Part print with two shaded views. Sizes in mm from the minimum x, y, z corner. A direction names the side the tool comes from. Round coordinates to 2 decimals unless told otherwise and drop trailing zeros. Loops run counter-clockwise (first coordinate to the right, second up) from the corner with the lowest first, then second, coordinate; pieces in that order, holes last. Notation, with made-up numbers: (17, 7) - (66, 7) arc R9 cw to (66, 22) - close; hole circle Ø3 at (85.25, -0.75). An arc over 180 degrees is marked (long way). Use a Markdown table: item, result.
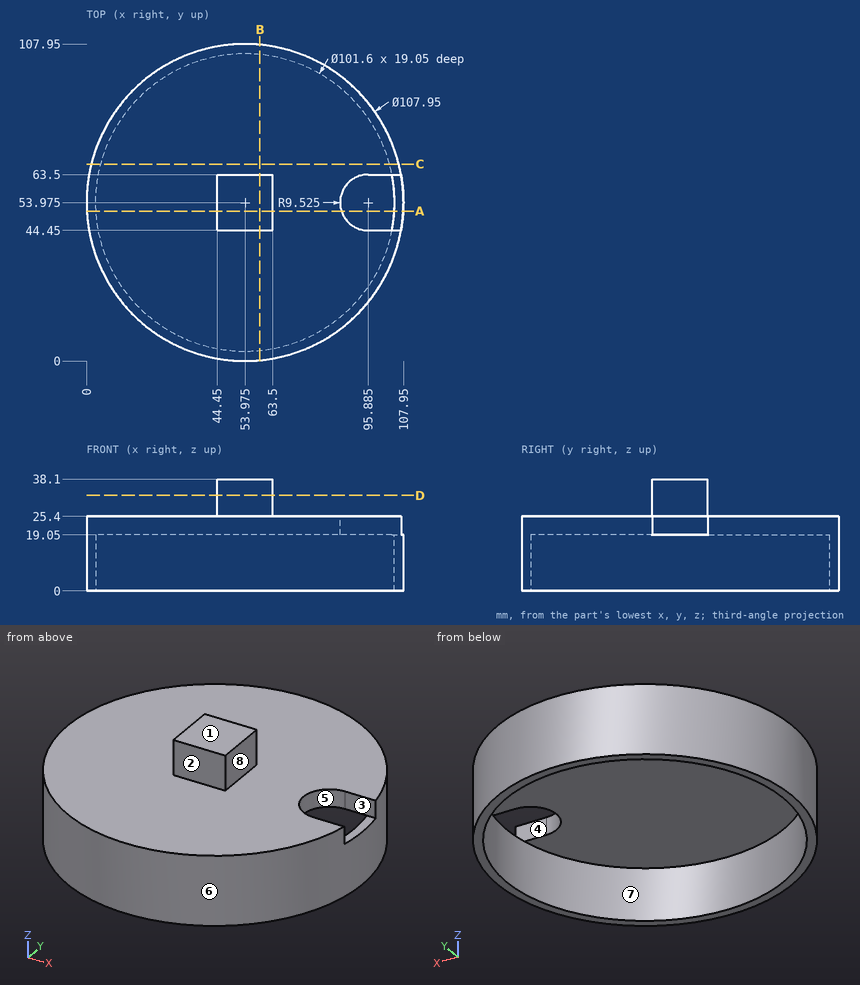
Q1. Which spindle directions (+Z, -Z, +X, -X, +Y, -Y) get a long thin tool onto all of the face, cutting with end or side? Do the marked faces 4, 5, 6, 7 and 8. Say none if no direction does.
Results found:
| item | result |
|---|---|
| face 4 | +Z, +X |
| face 5 | +Z, -Z, +X |
| face 6 | +Z, -Z |
| face 7 | -Z |
| face 8 | +Z, +X, +Y, -Y |
Q2. Cut at A-A, the plane y = 51. List the corners of the cut face in (x, z).
Results found:
| item | result |
|---|---|
| outline | (0.08, 0) - (3.26, 0) - (3.26, 19.05) - (86.84, 19.05) - (86.84, 25.4) - (63.5, 25.4) - (63.5, 38.1) - (44.45, 38.1) - (44.45, 25.4) - (0.08, 25.4) - close; (104.69, 0) - (107.87, 0) - (107.87, 19.05) - (104.69, 19.05) - close |
Q3. Cut at B-B, the plane x = 59. List the corners of the cut face in (y, z), plus the area to 3 significant figures.
Results found:
| item | result |
|---|---|
| outline | (0.23, 0) - (3.42, 0) - (3.42, 19.05) - (104.53, 19.05) - (104.53, 0) - (107.72, 0) - (107.72, 25.4) - (63.5, 25.4) - (63.5, 38.1) - (44.45, 38.1) - (44.45, 25.4) - (0.23, 25.4) - close |
| area | 1,050 mm2 |
Q4. Cut at D-D, the plane z = 32.5. List the corners of the cut face in (x, y), plus the area to 3 significant figures.
Results found:
| item | result |
|---|---|
| outline | (44.45, 44.45) - (63.5, 44.45) - (63.5, 63.5) - (44.45, 63.5) - close |
| area | 363 mm2 |
Q5. Cut at C-C, the plane y = 67. List the corners of the cut face in (x, z).
Results found:
| item | result |
|---|---|
| outline | (1.6, 0) - (4.87, 0) - (4.87, 19.05) - (103.08, 19.05) - (103.08, 0) - (106.35, 0) - (106.35, 25.4) - (1.6, 25.4) - close |
Q6. Drop flat-ended pins along their axis: pin 1 (1.5 mm diameter, centred on x = 67, y = 65.5, fed in from +Z); pin 2 (10 mm diameter, centred on x = 57.5, z = 29.5, fed in from +Y); pin 3 (4 mm diameter, centred on y = 56.5, z = 31, fed in from -X). Give the stop position or say it passes through.
Results found:
| item | result |
|---|---|
| pin 1 | stops at z = 25.4 |
| pin 2 | stops at y = 107.95 |
| pin 3 | stops at x = 44.45 |
Q7. Pull direction Y, two halves, no side cores. Call the marked faces 1, 2 and 3: pulls with the +Y half, pulls with the -Y half, needs draft (parallel to the pull), parting line crosses it, or undercut.
Results found:
| item | result |
|---|---|
| face 1 | needs draft |
| face 2 | pulls with the -Y half |
| face 3 | undercut |
Q8. Probe line 1 (Z direction, x = 62, y = 9); line 2 (Y direction, x = 7.5, z = 18); line 3 (Y direction, x = 64, z = 16.5). List the from-to ranges inside material, lowest first.
Results found:
| item | result |
|---|---|
| line 1 | z = 19.05 to 25.4 |
| line 2 | y = 26.53 to 33.46, 74.49 to 81.42 |
| line 3 | y = 0.94 to 4.17, 103.78 to 107.01 |
